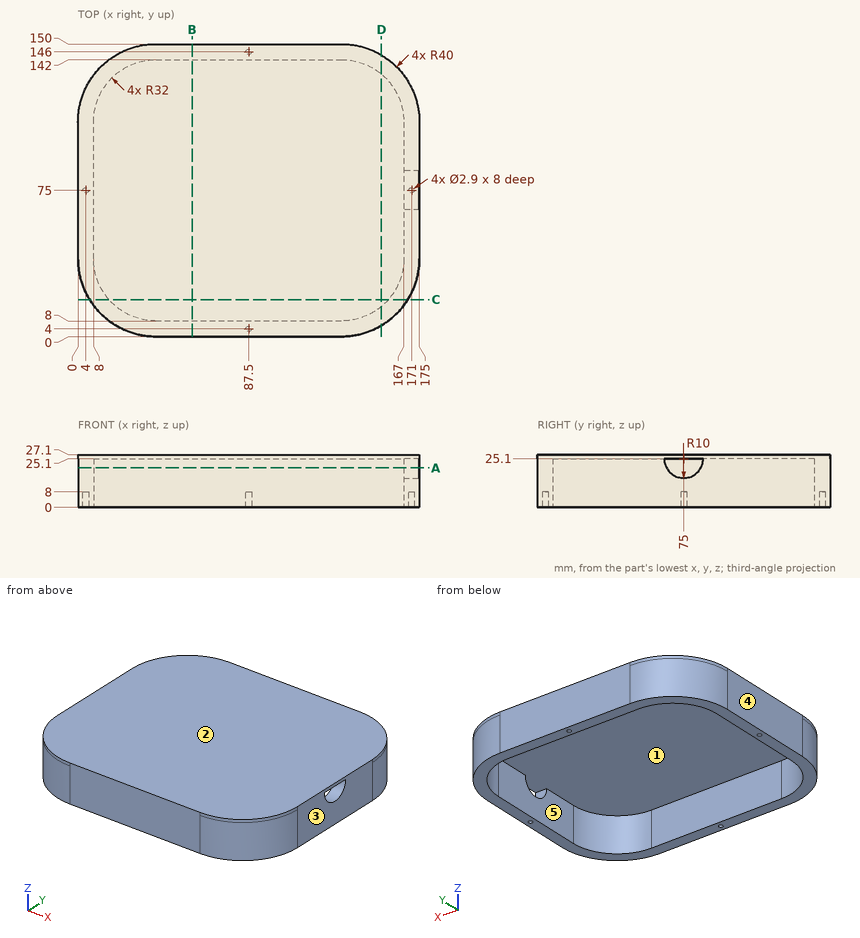
Geometry: see drawing. Coordinates: mm, zero at the bounding-box minimum. A direction names the side the tool comes from. Coordinates: 2 decimals unless noted, no trailing zeros. Loops run counter-clockwise (first coordinate to the right, second up) from the corner with the lowest first, then second, coordinate; pieces in that order, holes last. Notation, with made-up numbers: (39, 3) - (55, 3) arc R23 cw to (55, 35) - close; hole circle Ø11 at (-27.5, 36). An arc over 180 degrees is marked (long way). Put each result on its own line as item: value. Start each with the question number.
Q1. Pull-direction query (X, two-part tool) for the marked faces 1, 2 and 3; classes: released by +X, released by -X, zero draft, split by the parting line, or undercut.
Q2. Cut plane D-D, the plane x = 155.5. Return loops of the section in (y, z), and give its area (3 significant figures).
Q3. Cut plane C-C, the plane y = 19. Return loops of the section in (x, z), and give its area (3 significant figures).
Q4. Cut plane A-A, the plane z = 20.25. Return loops of the section in (x, y), and give its area (3 significant figures).
Q5. Pin query (flat end, axial travel): pin 1 Ø1.5 at (y, z) = (113, 7.5) entering from -X; pin 2 Ø8 at (x, z) = (149, 11.5) entering from +Y; pin 3 Ø0.9 at (x, y) = (87.5, 145.5) entering from -Z. Return the tip coordinate at first contact, or that it passes through.
Q6. Line query: line 1 (Y direction, x = 87.5, z = 2); line 2 (X direction, y = 75, z = 5.75); line 3 (Y direction, x = 86.5, z = 13). Output: solid intervals per line, ascending.
Q7. Cut plane B-B, the plane x = 58.5. Return loops of the section in (y, z).
Q8. Set-up query: the marked faces 4 and 5. Return all of +Z, -Z, +X, -X, +Y, -Y with unobstructed straight access to the full face (end or side cutting, diameter ignored); none if empty.
Filled sheet:
1. face 1: undercut
1. face 2: zero draft
1. face 3: released by +X
2. outline: (5.65, 0) - (15.43, 0) - (15.43, 25.1) - (134.57, 25.1) - (134.57, 0) - (144.35, 0) - (144.35, 27.1) - (5.65, 27.1) - close
2. area: 768 mm²
3. outline: (5.96, 0) - (15.85, 0) - (15.85, 25.1) - (159.15, 25.1) - (159.15, 0) - (169.04, 0) - (169.04, 27.1) - (5.96, 27.1) - close
3. area: 823 mm²
4. outline: (0, 40) arc R40 ccw to (40, 0) - (135, 0) arc R40 ccw to (175, 40) - (175, 66.25) - (167, 66.25) - (167, 40) arc R32 cw to (135, 8) - (40, 8) arc R32 cw to (8, 40) - (8, 110) arc R32 cw to (40, 142) - (135, 142) arc R32 cw to (167, 110) - (167, 83.75) - (175, 83.75) - (175, 110) arc R40 ccw to (135, 150) - (40, 150) arc R40 ccw to (0, 110) - close
4. area: 4,310 mm²
5. pin 1: x = 0.06
5. pin 2: y = 148.73
5. pin 3: z = 8
6. line 1: 0 to 2.55, 5.45 to 8, 142 to 144.55, 147.45 to 150
6. line 2: 0 to 2.55, 5.45 to 8, 167 to 169.55, 172.45 to 175
6. line 3: 0 to 8, 142 to 150
7. outline: (0, 0) - (8, 0) - (8, 25.1) - (142, 25.1) - (142, 0) - (150, 0) - (150, 27.1) - (0, 27.1) - close
8. face 4: +Z, -Z, -X, +Y, -Y
8. face 5: -Z
